Check sheet for the modelled part. Datum: model origin and axes. Units: mm. Coordinates: 2 decimals unless noted, no trailing zeros. Order: outer loops, then holes, each group sorted by start corner. A loop starts at its lowest first (then second) coordinate and runs counter-clockwise, first axis right, second up.
1. Cross-section at D-D (z = 1). Enter the section's corners in (x, y).
2. Draft check along Y on faces 1 (the flat face through (3, -5, 11.5)), 2 (the cylindrical face through (-1.19, -5.37, 9.28)), 3 (the cylindrical face through (-1.73, -7.81, 10.74)). Enter one of: released by +Y, released by -Y, zero draft, split by the parting line, or undercut.
3. Cross-section at C-C (z = 10.5). Enter the section's corners in (x, y).
4. Thickness scan on line 1 (Y direction, x = 0, z = 9); line 2 (X direction, y = -3.5, z = 4.25); line 3 (Y direction, x = 2.25, z = 4.5). Record the ranges inside material, lowest first.
5. Cross-section at A-A (x = 0). Enter the section's corners in (y, z), then the cut area to 3 significant figures.
6. Gauge pin test, flat ends, axial feed: pin 1 Ø2 at (x, y) = (-0.5, 1.5) entering from -Z; pin 2 Ø1.5 at (y, z) = (6, 6) entering from +X; pin 3 Ø3 at (y, z) = (-1, 2.5) entering from -X. Record the tip position at first contact, or that the pin passes through.
```python
from build123d import *

# Parameters (mm, degrees)
SKETCH2_R           = 7
BOSS_EXTRUDE1_DEPTH = 10
SKETCH3_R           = 8
BOSS_EXTRUDE2_DEPTH = 1.5
FILLET3_R           = 7
FILLET4_R           = 0.25


# Read off the part's stored shape, not the designer's step: Shell1
with BuildPart() as part:
    # Sketch2 → Boss-Extrude1 (new body)
    with BuildSketch(Plane.XY):
        Circle(SKETCH2_R)
    extrude(amount=BOSS_EXTRUDE1_DEPTH)

    # Sketch3 → Boss-Extrude2 (add)
    with BuildSketch(Plane.XY.offset(10)):
        Circle(SKETCH3_R)
    extrude(amount=BOSS_EXTRUDE2_DEPTH)

    # Fillet3
    fillet3_edges = [part.edges().sort_by_distance(p)[0] for p in [
        (-7, 0, 0),
    ]]
    fillet(fillet3_edges, radius=FILLET3_R)

    # Shell1 outline → Shell1 (revolve, cut)
    with BuildSketch(Plane.XZ):
        with BuildLine():
            Line((5.5, 7.000000005), (5.5, 11.5))
            Line((5.5, 11.5), (0, 11.5))
            Line((0, 11.5), (0, 1.5))
            ThreePointArc((0, 1.5), (3.889087298, 3.110912705), (5.5, 7.000000005))
        make_face()
    revolve(axis=Axis((0, 0, 0), (0, 0, 1)), mode=Mode.SUBTRACT)

    # Fillet4
    fillet4_edges = [part.edges().sort_by_distance(p)[0] for p in [
        (-8, 0, 10),
        (-8, 0, 11.5),
    ]]
    fillet(fillet4_edges, radius=FILLET4_R)


solid = part.part
```
Data:
1. outline: circle Ø7.21 at (0, 0)
2. face 1: zero draft
2. face 2: undercut
2. face 3: split by the parting line
3. outline: circle Ø16 at (0, 0); hole circle Ø11 at (0, 0)
4. line 1: y = -7 to -5.5, 5.5 to 7
4. line 2: x = -5.4 to -3.23, 3.23 to 5.4
4. line 3: y = -6.14 to -4.35, 4.35 to 6.14
5. outline: (-8, 10.25) arc R0.25 ccw to (-7.75, 10) - (-7, 10) - (-7, 7) arc R7 ccw to (7, 7) - (7, 10) - (7.75, 10) arc R0.25 ccw to (8, 10.25) - (8, 11.25) arc R0.25 ccw to (7.75, 11.5) - (5.5, 11.5) - (5.5, 7) arc R5.5 cw to (-5.5, 7) - (-5.5, 11.5) - (-7.75, 11.5) arc R0.25 ccw to (-8, 11.25) - close
5. area: 45.9 mm2
6. pin 1: stops at z = 0.02
6. pin 2: stops at x = 4.53
6. pin 3: stops at x = -6.27
